Source: CAD feature listing. Evaluate the final solid. Frame: model axes, mm. Round coordinates to 2 decimals unless told otherwise and drop trailing zeros. Order: outer loops, then holes, each group sorted by start corner. A loop starts at its lowest first (then second) coordinate and runs counter-clockwise, first axis right, second up. Notation, with made-up numbers: M 61,70.25 L 68,70.25 A9 ccw 68,81.25 Z; hole C 86.25,38.5 d2. An arc over 180 degrees is marked long. Answer in a Markdown table with one row per item. Add a question column.
```python
from build123d import *

# Parameters (mm, degrees)
F1_DEPTH = 25.4


with BuildPart() as f1:
    # F0 (on Front) → F1 (new body)
    with BuildSketch(Plane.XZ):
        with BuildLine():
            ThreePointArc((74.179427, -17.43137), (75.693171, -8.774044), (76.2, 0))
            ThreePointArc((76.2, 0), (75.693171, 8.774044), (74.179427, 17.43137))
            ThreePointArc((74.179427, 17.43137), (66.431298, 21.584837), (70.258319, 29.499298))
            ThreePointArc((70.258319, 29.499298), (61.647095, 44.789236), (49.766515, 57.703848))
            ThreePointArc((49.766515, 57.703848), (41.0568, 56.509837), (39.500921, 65.162238))
            ThreePointArc((39.500921, 65.162238), (23.547095, 72.470507), (6.344485, 75.935417))
            ThreePointArc((6.344485, 75.935417), (0, 69.85), (-6.344485, 75.935417))
            ThreePointArc((-6.344485, 75.935417), (-23.547095, 72.470507), (-39.500921, 65.162238))
            ThreePointArc((-39.500921, 65.162238), (-38.710449, 63.483083), (-38.439236, 61.647095))
            ThreePointArc((-38.439236, 61.647095), (-42.70156, 55.650087), (-49.766515, 57.703848))
            ThreePointArc((-49.766515, 57.703848), (-61.647095, 44.789236), (-70.258319, 29.499298))
            ThreePointArc((-70.258319, 29.499298), (-67.256588, 27.171671), (-66.120507, 23.547095))
            ThreePointArc((-66.120507, 23.547095), (-68.631831, 18.488728), (-74.179427, 17.43137))
            ThreePointArc((-74.179427, 17.43137), (-76.2, 0), (-74.179427, -17.43137))
            ThreePointArc((-74.179427, -17.43137), (-68.631831, -18.488728), (-66.120507, -23.547095))
            ThreePointArc((-66.120507, -23.547095), (-67.256588, -27.171671), (-70.258319, -29.499298))
            ThreePointArc((-70.258319, -29.499298), (-61.647095, -44.789236), (-49.766515, -57.703848))
            ThreePointArc((-49.766515, -57.703848), (-42.70156, -55.650087), (-38.439236, -61.647095))
            ThreePointArc((-38.439236, -61.647095), (-38.710449, -63.483083), (-39.500921, -65.162238))
            ThreePointArc((-39.500921, -65.162238), (-23.547095, -72.470507), (-6.344485, -75.935417))
            ThreePointArc((-6.344485, -75.935417), (0, -69.85), (6.344485, -75.935417))
            ThreePointArc((6.344485, -75.935417), (23.547095, -72.470507), (39.500921, -65.162238))
            ThreePointArc((39.500921, -65.162238), (41.0568, -56.509837), (49.766515, -57.703848))
            ThreePointArc((49.766515, -57.703848), (61.647095, -44.789236), (70.258319, -29.499298))
            ThreePointArc((70.258319, -29.499298), (66.431298, -21.584837), (74.179427, -17.43137))
        make_face()
    extrude(amount=F1_DEPTH)


solid = f1.part
```
(1) Pin query (flat end, axial travel): pin 1 (6 mm diameter, centred on y = -22.5, z = -27, fed in from +X); pin 2 (10 mm diameter, centred on x = 60.5, y = -20.5, fed in from +Z); pin 3 (1.5 mm diameter, centred on x = 26.5, y = -8.5, fed in from -Z); pin 4 (12 mm diameter, centred on x = -1, z = -19.5, fed in from +Y). Return the tip coordinate at first contact, or that it passes through.
(2) Cut plane B-B (x = 0). Return loops of the section in (y, z).
(3) Draft query along X for faces 1 (the face through (40.95, -12.52, -56.59)), 2 (the face through (-76.2, -12.5, 0.2)), 3 (the face through (23.313, -12.522, -72.546)), 4 (the face through (-0.14, -12.52, -69.85)). Return one class per face: +X half, -X half, draft (parallel to the pull), parting line (faces both ways), or undercut.
(4) Cut plane C-C (z = -53.5). Return loops of the section in (x, y), and give its area (3 significant figures).
(5) Cut plane A-A (y = -15). Return loops of the section in (x, z).
(6) Line query: line 1 (X direction, y = -11.75, z = -39.5); line 2 (X direction, y = -8, z = 57); line 3 (X direction, y = -6.25, z = -2). Output: solid intervals per line, ascending. Write a range as from..to.
Answer list:
| question | item | result |
|---|---|---|
| 1 | pin 1 | x = 70.26 |
| 1 | pin 2 | z = 52.21 |
| 1 | pin 3 | z = -71.72 |
| 1 | pin 4 | y = 0 |
| 2 | outline | M -25.4,-69.85 L 0,-69.85 L 0,69.85 L -25.4,69.85 Z |
| 3 | face 1 | undercut |
| 3 | face 2 | -X half |
| 3 | face 3 | +X half |
| 3 | face 4 | undercut |
| 4 | outline | M -54.26,-25.4 L 54.26,-25.4 L 54.26,0 L -54.26,0 Z |
| 4 | area | 2,760 mm² |
| 5 | outline | M -74.18,-17.43 A6.35 cw -66.12,-23.55 A6.35 cw -70.26,-29.5 A76.2 ccw -49.77,-57.7 A6.35 cw -39.5,-65.16 A76.2 ccw -6.34,-75.94 A6.35 cw 6.34,-75.94 A76.2 ccw 39.5,-65.16 A6.35 cw 49.77,-57.7 A76.2 ccw 70.26,-29.5 A6.35 cw 74.18,-17.43 A76.2 ccw 76.2,0 A76.2 ccw 74.18,17.43 A6.35 cw 70.26,29.5 A76.2 ccw 49.77,57.7 A6.35 cw 39.5,65.16 A76.2 ccw 6.34,75.94 A6.35 cw -6.34,75.94 A76.2 ccw -39.5,65.16 A6.35 cw -49.77,57.7 A76.2 ccw -70.26,29.5 A6.35 cw -66.12,23.55 A6.35 cw -74.18,17.43 A76.2 ccw Z |
| 6 | line 1 | -65.16..65.16 |
| 6 | line 2 | -50.57..-49.12, -40.46..40.46, 49.12..50.57 |
| 6 | line 3 | -76.17..76.17 |
